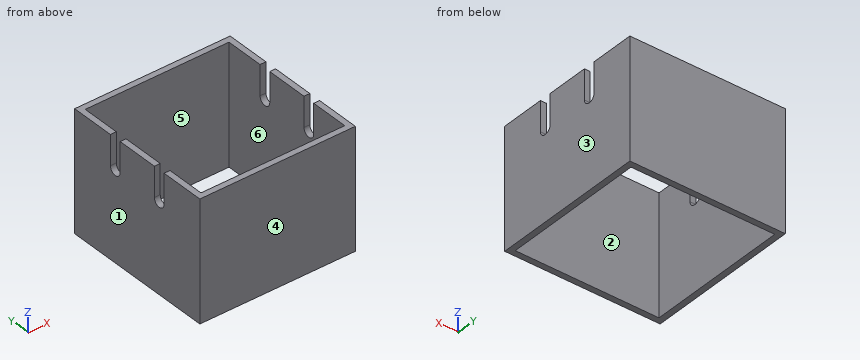
```python
from build123d import *

# Parameters (mm, degrees)
SKETCH1_W           = 130
SKETCH1_H           = 130
BOSS_EXTRUDE1_DEPTH = 100
SKETCH2_W           = 120.2
SKETCH2_H           = 120.2
CUT_EXTRUDE1_DEPTH  = 1000
CUT_EXTRUDE2_DEPTH  = 1000


with BuildPart() as part:
    # Sketch1 → Boss-Extrude1 (new body)
    with BuildSketch(Plane(origin=(0, 0, 0), x_dir=(0, 1, 0), z_dir=(0, 0, 1))):
        Rectangle(SKETCH1_W, SKETCH1_H)
    extrude(amount=BOSS_EXTRUDE1_DEPTH)

    # Sketch2 → Cut-Extrude1 (cut)
    with BuildSketch(Plane.XY.offset(100)):
        Rectangle(SKETCH2_W, SKETCH2_H)
    extrude(amount=-CUT_EXTRUDE1_DEPTH, mode=Mode.SUBTRACT)

    # Sketch3 → Cut-Extrude2 (cut)
    with BuildSketch(Plane(origin=(-65, 0, 0), x_dir=(0, -1, 0), z_dir=(-1, 0, 0))):
        with BuildLine():
            Line((27.875, 100), (17.775, 100))
            Line((17.775, 100), (17.775, 75))
            ThreePointArc((17.775, 75), (22.825, 80.05), (27.875, 75))
            Line((27.875, 75), (27.875, 100))
        make_face()
        with BuildLine():
            Line((-17.775, 100), (-27.875, 100))
            Line((-27.875, 100), (-27.875, 75))
            ThreePointArc((-27.875, 75), (-22.825, 80.05), (-17.775, 75))
            Line((-17.775, 75), (-17.775, 100))
        make_face()
        with BuildLine():
            ThreePointArc((-17.775, 75), (-22.825, 80.05), (-27.875, 75))
            Line((-27.875, 75), (-17.775, 75))
        make_face()
        with BuildLine():
            Line((-17.775, 75), (-27.875, 75))
            ThreePointArc((-27.875, 75), (-22.825, 69.95), (-17.775, 75))
        make_face()
        with BuildLine():
            ThreePointArc((27.875, 75), (22.825, 80.05), (17.775, 75))
            Line((17.775, 75), (27.875, 75))
        make_face()
        with BuildLine():
            Line((27.875, 75), (17.775, 75))
            ThreePointArc((17.775, 75), (22.825, 69.95), (27.875, 75))
        make_face()
    extrude(amount=-CUT_EXTRUDE2_DEPTH, mode=Mode.SUBTRACT)


solid = part.part
```
Read the model definition and answer for the solid it produces. Units are mm, in the model's axes. Face numbers are marked on the shaded views. A direction names the side the tool comes from. Round coordinates to 2 decimals unless told otherwise and drop trailing zeros. Write each loop counter-clockwise with the first axis right and the second up, starting at its lowest first coordinate (ties: lowest second). Pieces come first, ordered by that corner, then holes. Notation, with made-up numbers: (78, -24) - (123, -24) arc R15 ccw to (123, -17) - close; hole circle Ø7 at (61.25, -9). An arc over 180 degrees is marked (long way). One line per item, written item: value.
Q1. Find section D-D (z = 73). Determine the outline of the cut face in (x, y).
The answers:
outline: (-65, -65) - (65, -65) - (65, -27.46) - (60.1, -27.46) - (60.1, -60.1) - (-60.1, -60.1) - (-60.1, -27.46) - (-65, -27.46) - close; (-65, -18.19) - (-60.1, -18.19) - (-60.1, 18.19) - (-65, 18.19) - close; (-65, 27.46) - (-60.1, 27.46) - (-60.1, 60.1) - (60.1, 60.1) - (60.1, 27.46) - (65, 27.46) - (65, 65) - (-65, 65) - close; (60.1, -18.19) - (65, -18.19) - (65, 18.19) - (60.1, 18.19) - close
Q2. Find section A-A (y = 3.5). Determine the outline of the cut face in (x, z).
The answers:
outline: (-65, 0) - (-60.1, 0) - (-60.1, 100) - (-65, 100) - close; (60.1, 0) - (65, 0) - (65, 100) - (60.1, 100) - close
Q3. Which of the six approach directions +Z, -Z, +X, -X, +Y, -Y give full straight-line access (tool end or side, diameter ignored) to the marked faces 1 and 2?
The answers:
face 1: +Z, -Z, -X, +Y, -Y
face 2: +Z, -Z
Q4. A straight line is drawn through the part: line 1 (X direction, y = -50, z = 25). Find the intervals that lie inside material, in ascending order. Write a range as from..to.
The answers:
line 1: x = -65..-60.1, 60.1..65
Q5. For a pull along X with two mould halves and no side action, classify the marked faces 3, 4, 5 and 6 as pulls with the +X half, pulls with the -X half, needs draft (parallel to the pull), parting line crosses it, or undercut.
The answers:
face 3: pulls with the +X half
face 4: needs draft
face 5: undercut
face 6: undercut
Q6. Find section C-C (z = 9). Determine the outline of the cut face in (x, y), and give its area (3 significant figures).
The answers:
outline: (-65, -65) - (65, -65) - (65, 65) - (-65, 65) - close; hole (-60.1, -60.1) - (60.1, -60.1) - (60.1, 60.1) - (-60.1, 60.1) - close
area: 2,450 mm2
